Autodesk Inventor part; units mm, degrees
ref_plane "YZ Plane" through (0, 0, 0) normal (1, 0, 0) x (0, 1, 0)
ref_plane "XZ Plane" through (0, 0, 0) normal (0, 1, 0) x (-1, 0, 0)
ref_plane "XY Plane" through (0, 0, 0) normal (0, 0, 1) x (1, 0, 0)
sketch "Sketch1" plane through (0, 0, 0) normal (0, 0, 1) x (1, 0, 0)
  line L0 (-30, 10) -> (30, 10)
  line L1 (30, 10) -> (30, -10)
  line L2 (30, -10) -> (-30, -10)
  line L3 (-30, -10) -> (-30, 10)
  line L4 (-30, 10) -> (30, -10) construction
  line L5 (30, 10) -> (-30, -10) construction
  circle A0 centre (18, 0) radius 3.5
  circle A1 centre (-18, 0) radius 3.5
  line L6 (0, 10) -> (0, -10) construction
  point P0 (0, 0)
  point P1 (0, 0)
  dimension "d0" = 60
  dimension "d1" = 20
  dimension "d2" = 7
  dimension "d3" = 36
extrude "Plate1" add sketch "Sketch1" along normal blind 2
fillet "Corner Round1" radius 6 4 edges at (-30, 10, 1) (-30, -10, 1) (30, 10, 1) (30, -10, 1)
equation "\"d4\" = Thickness"
equation "\"BendRadius\" = Thickness"
equation "\"BendReliefWidth\" = Thickness"
equation "\"BendReliefDepth\" = 0.5 * Thickness"
equation "\"CornerReliefSize\" = 4 * Thickness"
equation "\"MinimumRemnant\" = 2 * Thickness"
equation "\"TransitionRadius\" = BendRadius"
equation "\"JacobiRadiusSize\" = BendRadius"
equation "\"GapSize\" = Thickness"
properties part number "motor pillar 1"
Could you check a few things on this model? Use its own coordinates, in mm. Coordinates: 2 decimals unless noted, no trailing zeros. Write each loop counter-clockwise with the first axis right and the second up, starting at its lowest first coordinate (ties: lowest second). Pieces come first, ordered by that corner, then holes. Notation, with made-up numbers: (-10, 3) -> (13, 3) arc R11 cw to (13, 17) -> close; hole circle Ø1 at (30, -21.5). An arc over 180 degrees is marked (long way). Return JSON: item names as keys, results as strings.
(1) Imagine slicing it at B-B, the plane z = 1.4. Please give me the cut outline in (x, y).
Numbers:
{"outline": "(-30, -4) arc R6 ccw to (-24, -10) -> (24, -10) arc R6 ccw to (30, -4) -> (30, 4) arc R6 ccw to (24, 10) -> (-24, 10) arc R6 ccw to (-30, 4) -> close; hole circle Ø7 at (-18, 0); hole circle Ø7 at (18, 0)"}
(2) Imagine slicing it at D-D, the plane y = 2.75. Please give me the cut outline in (x, z).
Numbers:
{"outline": "(-30, 0) -> (-20.17, 0) -> (-20.17, 2) -> (-30, 2) -> close; (-15.83, 0) -> (15.83, 0) -> (15.83, 2) -> (-15.83, 2) -> close; (20.17, 0) -> (30, 0) -> (30, 2) -> (20.17, 2) -> close"}
(3) I'm going to push a flat-ended pin straight in: pin 1 (5.5 mm diameter, centred on x = -18, y = 0, fed in from +Z). Where does the tip first touch, or does it pass through?
Numbers:
{"pin 1": "passes through"}
(4) I need wall thicknesses on L1, parallel to Y at x = -18, z = 0.8; L2, parallel to X at y = -1.5, z = 0.6; L3, parallel to X at y = -1, z = 0.65. Which ranges of each line are inside material? Lowest first, please.
Numbers:
{"L1": "y = -10 to -3.5, 3.5 to 10", "L2": "x = -30 to -21.16, -14.84 to 14.84, 21.16 to 30", "L3": "x = -30 to -21.35, -14.65 to 14.65, 21.35 to 30"}
(5) Imagine slicing it at A-A, the plane x = -18. Please give me the cut outline in (y, z).
Numbers:
{"outline": "(-10, 0) -> (-3.5, 0) -> (-3.5, 2) -> (-10, 2) -> close; (3.5, 0) -> (10, 0) -> (10, 2) -> (3.5, 2) -> close"}
(6) Imagine slicing it at C-C, the plane y = 0. Please give me the cut outline in (x, z), then the cut area to 3 significant figures.
Numbers:
{"outline": "(-30, 0) -> (-21.5, 0) -> (-21.5, 2) -> (-30, 2) -> close; (-14.5, 0) -> (14.5, 0) -> (14.5, 2) -> (-14.5, 2) -> close; (21.5, 0) -> (30, 0) -> (30, 2) -> (21.5, 2) -> close", "area": "92.0 mm2"}
(7) We'd pull the mould along Y, two halves only. Please class faces 1 (the flat face through (0, 10, 1)), 2 (the flat face through (0, -10, 1)), 3 (the flat face through (0, 0, 2)), 4 (the cylindrical face through (21.34, -1.05, 0.99)): +Y half, -Y half, draft (parallel to the pull), parting line (faces both ways), or undercut.
Numbers:
{"face 1": "+Y half", "face 2": "-Y half", "face 3": "draft", "face 4": "undercut"}
